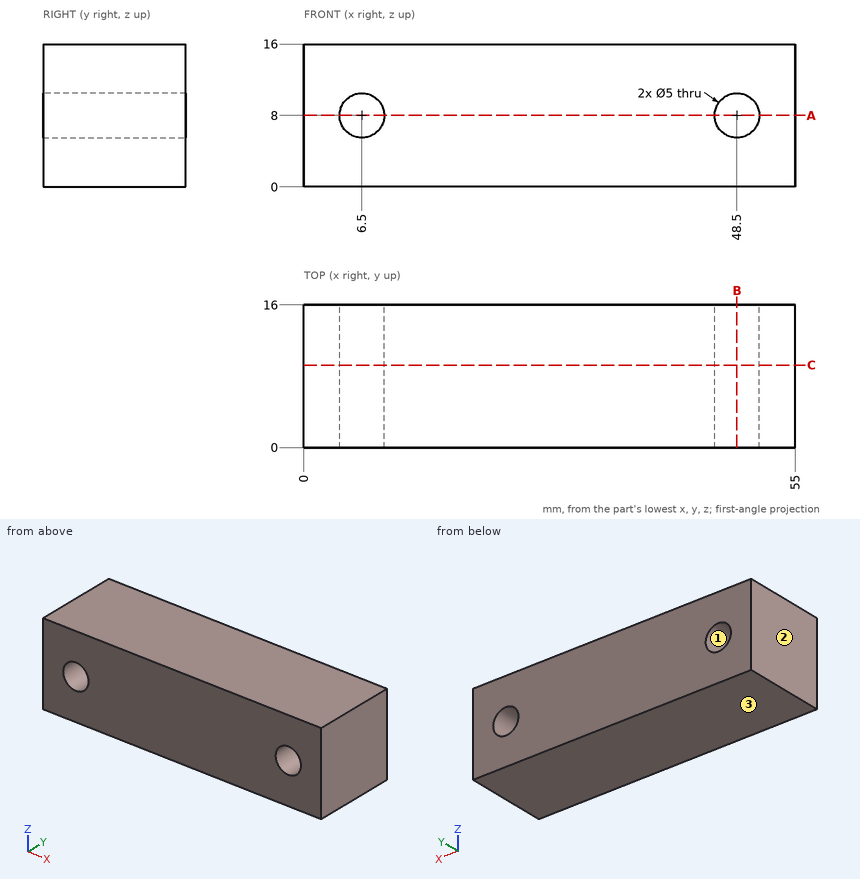
The drawing under review shows one solid part. Ordinate dimensions are in mm from its lowest x, y, z. Round coordinates to 2 decimals unless told otherwise and drop trailing zeros. Write each loop counter-clockwise with the first axis right and the second up, starting at its lowest first coordinate (ties: lowest second). Pieces come first, ordered by that corner, then holes. Notation, with made-up numbers: (-18.5, -32) - (11.5, -32) arc R23 ccw to (11.5, -14) - close; hole circle Ø7 at (-10, -28.75). An arc over 180 degrees is marked (long way). Put each result on its own line as item: value.
Q1. We need section A-A (z = 8). Give the boundary of the cut face in (x, y).
Solved:
outline: (0, 0) - (4, 0) - (4, 16) - (0, 16) - close; (9, 0) - (46, 0) - (46, 16) - (9, 16) - close; (51, 0) - (55, 0) - (55, 16) - (51, 16) - close
Q2. Insertion check: pin 1 Ø4 at (x, z) = (6.5, 8) entering from -Y. The pin has a flat end and moves straight along its axis. Give the tip position at first contact, or say it passes through.
Solved:
pin 1: passes through
Q3. We need section B-B (x = 48.5). Give the boundary of the cut face in (y, z), and give its area (3 significant figures).
Solved:
outline: (0, 0) - (16, 0) - (16, 5.5) - (0, 5.5) - close; (0, 10.5) - (16, 10.5) - (16, 16) - (0, 16) - close
area: 176 mm2
Q4. Wall thickness on probe 1 along X at (y, z) = (10, 8); probe 2 along X at (y, z) = (6, 7.5); probe 3 along Z at (x, y) = (49, 10): over which ranges is each line inside the solid? List them lowest first.
Solved:
probe 1: x = 0 to 4, 9 to 46, 51 to 55
probe 2: x = 0 to 4.05, 8.95 to 46.05, 50.95 to 55
probe 3: z = 0 to 5.55, 10.45 to 16
Q5. Mouldability with a two-part tool opening along X and no side actions: class the marked faces 1, 2 and 3 as released by +X, released by -X, zero draft, split by the parting line, or undercut.
Solved:
face 1: undercut
face 2: released by -X
face 3: zero draft
Q6. We need section C-C (y = 9.25). Give the boundary of the cut face in (x, z).
Solved:
outline: (0, 0) - (55, 0) - (55, 16) - (0, 16) - close; hole circle Ø5 at (6.5, 8); hole circle Ø5 at (48.5, 8)
